from build123d import *

# Parameters (mm, degrees)
SKETCH1_W               = 2
SKETCH1_H               = 25
SKETCH2_W               = 0.5
SKETCH2_H               = 1.642734333
CUT_EXTRUDE1_DEPTH      = 4
CUT_EXTRUDE1_DEPTH_BACK = 4


with BuildPart() as part:
    # Sketch1 → Revolve1 (revolve)
    with BuildSketch(Plane.XY):
        with Locations((1, -12.5)):
            Rectangle(SKETCH1_W, SKETCH1_H)
        with BuildLine():
            Line((0, 0), (3, 0))
            ThreePointArc((3, 0), (2.121320344, 2.121320344), (0, 3))
            Line((0, 3), (0, 0))
        make_face()
    revolve(axis=Axis((0, 3, 0), (0, -1, 0)))

    # Sketch2 → Cut-Extrude1 (cut, two sides)
    with BuildSketch(Plane.XY) as cut_extrude1_sk:
        with Locations((-0.25, 2.321367166)):
            Rectangle(SKETCH2_W, SKETCH2_H)
        with Locations((0.25, 2.321367166)):
            Rectangle(SKETCH2_W, SKETCH2_H)
    extrude(amount=CUT_EXTRUDE1_DEPTH, mode=Mode.SUBTRACT)
    extrude(cut_extrude1_sk.sketch, amount=-CUT_EXTRUDE1_DEPTH_BACK, mode=Mode.SUBTRACT)


solid = part.part
Could you check a few things on this model? Use its own coordinates, in mm. A direction names the side the tool comes from. Give positions to 0.01 mm unless a question says otherwise; leave off trailing zeros. Order: outer loops, then holes, each group sorted by start corner. A loop starts at its lowest first (then second) coordinate and runs counter-clockwise, first axis right, second up.
1. Suppose I cut it at C-C (y = -21). List the corners of the cut face in (x, z) for me.
2. Suppose I cut it at D-D (z = -1.6). List the corners of the cut face in (x, y) for me.
3. Will these pins go through, and if not, where does the flat tip stop? P1, Ø2, axis at x = -0.5, z = 2, coming from the +Y side; P2, Ø1.6, axis at y = 2.5, z = -0.5, coming from the +X side; P3, Ø0.8, axis at x = 0, z = -0.5, coming from the +Y side.
4. We'd pull the mould along X, two halves only. Please class faces 3 (the flat face through (0.5, 2, 0)), 4 (the cylindrical face through (0, -12, -2)), 5 (the flat face through (-1, 0, -2)): pulls with the +X half, pulls with the -X half, needs draft (parallel to the pull), parting line crosses it, or undercut.
5. For faces 1 (the flat face through (0, -25, 0)), 2 (the flat face through (0, 1.5, 0)), which set-ups out of +Z, -Z, +X, -X, +Y, -Y let a thin tool reach every point of the face, with its end or its side?
6. I need wall thicknesses on L1, parallel to Y at x = -0.35, z = 1.35; L2, parallel to Y at x = 0.15, z = -2.3; L3, parallel to X at y = -15, z = -0.05. Which ranges of each line are inside material? Lowest first, please.
7. Suppose I cut it at B-B (z = 0). List the corners of the cut face in (x, y) for me.
8. Suppose I cut it at A-A (x = 0). List the corners of the cut face in (y, z) for me.
Solved:
1. outline: circle Ø4 at (0, 0)
2. outline: (-2.54, 0) - (-1.2, 0) - (-1.2, -25) - (1.2, -25) - (1.2, 0) - (2.54, 0) arc R2.54 ccw to (0.5, 2.49) - (0.5, 1.5) - (-0.5, 1.5) - (-0.5, 2.49) arc R2.54 ccw to start
3. P1: stops at y = 2.78
3. P2: stops at x = 2.44
3. P3: stops at y = 1.5
4. face 3: undercut
4. face 4: parting line crosses it
4. face 5: needs draft
5. face 1: +Z, -Z, +X, -X, -Y
5. face 2: +Z, -Z, +Y
6. L1: y = -25 to 1.5
6. L2: y = 0 to 1.5
6. L3: x = -2 to 2
7. outline: (-3, 0) - (-2, 0) - (-2, -25) - (2, -25) - (2, 0) - (3, 0) arc R3 ccw to (0.5, 2.96) - (0.5, 1.5) - (-0.5, 1.5) - (-0.5, 2.96) arc R3 ccw to start
8. outline: (-25, -2) - (0, -2) - (0, -3) arc R3 ccw to (1.5, -2.6) - (1.5, 2.6) arc R3 ccw to (0, 3) - (0, 2) - (-25, 2) - close
